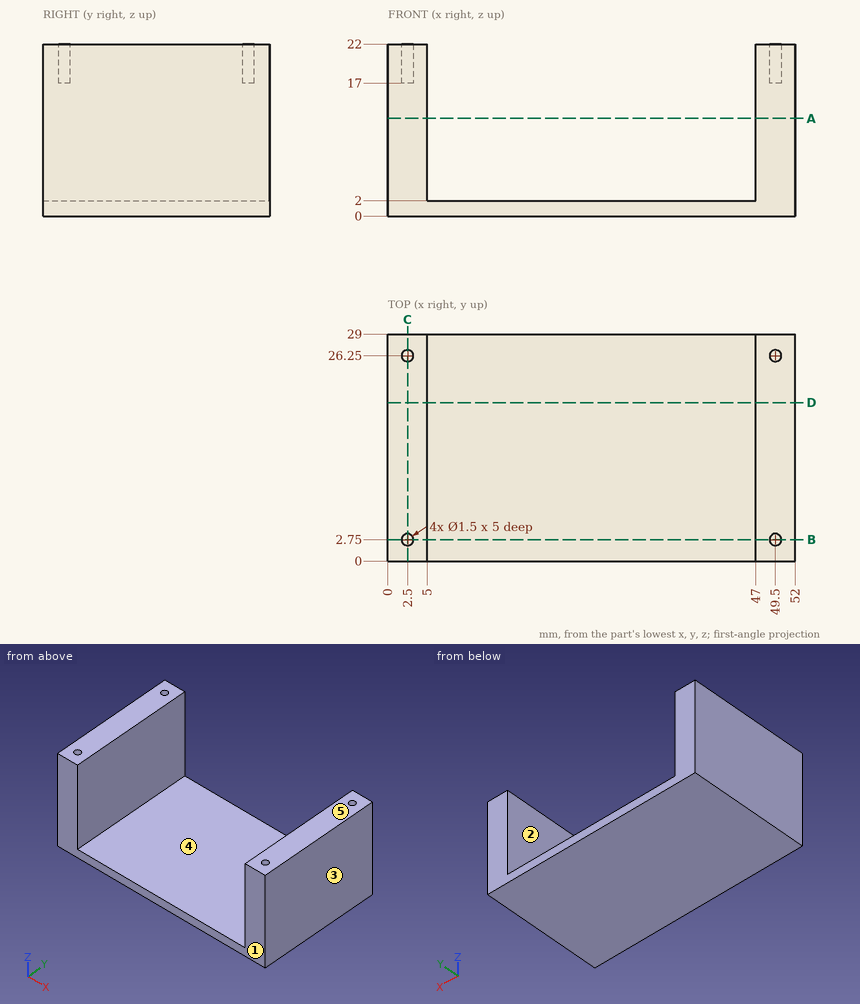
Part print with two shaded views. Sizes in mm from the minimum x, y, z corner. A direction names the side the tool comes from. Give positions to 0.01 mm unless a question says otherwise; leave off trailing zeros. Order: outer loops, then holes, each group sorted by start corner. A loop starts at its lowest first (then second) coordinate and runs counter-clockwise, first axis right, second up.
(1) Saw through at D-D, the plane y = 20.25. Give the cut face in (x, z).
(2) Saw through at B-B, the plane y = 2.75. Give the cut face in (x, z).
(3) Mould opens along X. For the marked faces 3, 4 and 5 say: released by +X, released by -X, zero draft, split by the parting line, or undercut.
(4) Tool access for the marked faces 1 and 2: list every direction of +Z, -Z, +X, -X, +Y, -Y with a clear straight run to the whole face (end or side of a thin tool).
(5) Drill centre lines: L1, parallel to Y at x = 2.5, z = 20.8; L2, parallel to X at y = 11.25, z = 6.25; L3, parallel to Z at x = 22.5, y = 7.75. Where is each one in solid material? Low to high.
(6) Saw through at A-A, the plane z = 12.5. Give the cut face in (x, y), then the cut area to 3 significant figures.
(7) Flat gauge pins, fed straight in: pin 1 (1.4 mm diameter, centred on x = 2.5, y = 26.25, fed in from +Z); pin 2 (1.5 mm diameter, centred on x = 37.5, y = 17, fed in from +Z). Where does each tip first touch, or does it go through?
(8) Saw through at C-C, the plane x = 2.5. Give the cut face in (y, z).
Results found:
1. outline: (0, 0) - (52, 0) - (52, 22) - (47, 22) - (47, 2) - (5, 2) - (5, 22) - (0, 22) - close
2. outline: (0, 0) - (52, 0) - (52, 22) - (50.25, 22) - (50.25, 17) - (48.75, 17) - (48.75, 22) - (47, 22) - (47, 2) - (5, 2) - (5, 22) - (3.25, 22) - (3.25, 17) - (1.75, 17) - (1.75, 22) - (0, 22) - close
3. face 3: released by +X
3. face 4: undercut
3. face 5: zero draft
4. face 1: +Z, -Z, +X, -X, -Y
4. face 2: +Z, +Y, -Y
5. L1: y = 0 to 2, 3.5 to 25.5, 27 to 29
5. L2: x = 0 to 5, 47 to 52
5. L3: z = 0 to 2
6. outline: (0, 0) - (5, 0) - (5, 29) - (0, 29) - close; (47, 0) - (52, 0) - (52, 29) - (47, 29) - close
6. area: 290 mm2
7. pin 1: stops at z = 17
7. pin 2: stops at z = 2
8. outline: (0, 0) - (29, 0) - (29, 22) - (27, 22) - (27, 17) - (25.5, 17) - (25.5, 22) - (3.5, 22) - (3.5, 17) - (2, 17) - (2, 22) - (0, 22) - close
